Can you work these out from the model? Positions are in its coordinate system, mm. A direction names the side the tool comes from. Round coordinates to 2 decimals unless told otherwise and drop trailing zeros. Loops run counter-clockwise (first coordinate to the right, second up) from the corner with the lowest first, then second, coordinate; pieces in that order, holes last. Notation, with made-up numbers: M 21,-10 L 28,-10 A25 cw 28,7 Z; hole C 9,-25 d11. An arc over 180 degrees is marked long. Answer as CSV lines item,"result".
Autodesk Inventor part; units mm, degrees
ref_plane "YZ Plane" through (0, 0, 0) normal (1, 0, 0) x (0, 1, 0)
ref_plane "XZ Plane" through (0, 0, 0) normal (0, 1, 0) x (-1, 0, 0)
ref_plane "XY Plane" through (0, 0, 0) normal (0, 0, 1) x (1, 0, 0)
sketch "Sketch1" plane through (0, 0, 0) normal (0, 0, 1) x (1, 0, 0)
  line L0 (0, 0) -> (25, 0)
  line L1 (25, 0) -> (25, 15)
  line L2 (25, 15) -> (5, 15)
  circle A0 centre (20, 5) radius 1.6
  line L3 (5, 10) -> (0, 10)
  line L4 (0, 10) -> (0, 0)
  line L5 (5, 10) -> (5, 15)
  dimension "d2" = 3.2
  dimension "d3" = 10
  dimension "d4" = 5
  dimension "d12" = 20
  dimension "d16" = 15
  dimension "d17" = 5
  dimension "d18" = 5
extrude "Extrusion1" add sketch "Sketch1" along normal blind 6.731
fillet "Fillet1" radius 5 1 edges at (25, 0, 3.3655)
equation "\"d18\" = d17"
equation "\"d6\" = THICKB"
equation "\"THICKA\" = 3.175"
equation "\"THICKB\" = 6.731"
equation "\"THICKC\" = 12.7"
equation "\"BALLDIA\" = 12"
equation "\"MAGDIA\" = 9.5"
properties part number "Carriage_Belt_Lock_Flap"
Item 1: We'd pull the mould along Y, two halves only. Please class faces 3 (the face through (3, 10, 3)), 4 (the face through (23, 1, 3)), 5 (the face through (18.82, 3.92, 3.32)), 6 (the face through (25, 10, 3)): released by +Y, released by -Y, zero draft, split by the parting line, or undercut.
Output:
face 3,"released by +Y"
face 4,"released by -Y"
face 5,"undercut"
face 6,"zero draft"
Item 2: If we section it at A-A on z = 2.75: Write out the boundary of the cut face in (x, y), then the cut area to 3 significant figures.
Output:
outline,"M 0,0 L 20,0 A5 ccw 25,5 L 25,15 L 5,15 L 5,10 L 0,10 Z; hole C 20,5 d3.2"
area,"337 mm2"
Item 3: If I drill on line 1 along Y through (x, z) = (20, 2.75); line 2 along X through (y, z) = (11, 2.25); line 3 along Y through (x, z) = (21, 3), over which ranges is the centre line in solid material (lowest first)? Write a range as from..to.
Output:
line 1,"y = 0..3.4, 6.6..15"
line 2,"x = 5..25"
line 3,"y = 0.1..3.75, 6.25..15"
Item 4: On a 3-axis mill with a long thin cutter (end or side, diameter ignored), from which of +Z, -Z, +X, -X, +Y, -Y can I reach the whole of each face in a straight line? I mean faces 1 (the face through (5, 12, 3)), 2 (the face through (12, 8, 0)). Say none if no direction works.
Output:
face 1,"+Z, -Z, -X, +Y"
face 2,"-Z, +X, -X, +Y, -Y"
Item 5: If we section it at B-B on y = 11: Write out the boundary of the cut face in (x, z), then the cut area to 3 significant figures.
Output:
outline,"M 5,0 L 25,0 L 25,6.73 L 5,6.73 Z"
area,"135 mm2"
Item 6: Will this pin go through, and if not, where does the flat tip stop? pin 1 (2.5 mm diameter, centred on y = 11.5, z = 2, fed in from -X).
Output:
pin 1,"stops at x = 5"
